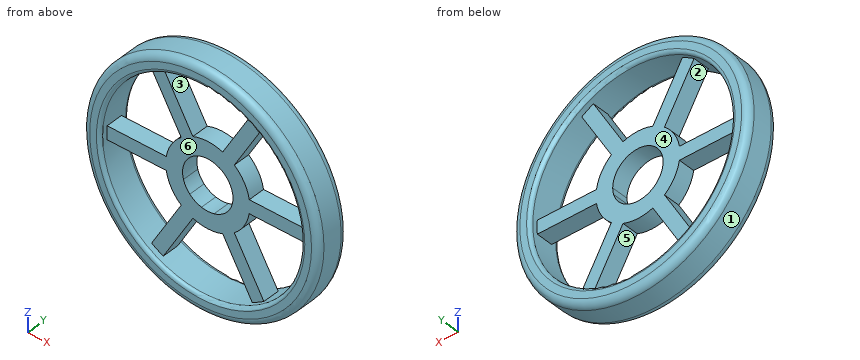
Autodesk Inventor part; units mm, degrees
ref_plane "YZ Plane" through (0, 0, 0) normal (1, 0, 0) x (0, 1, 0)
ref_plane "XZ Plane" through (0, 0, 0) normal (0, 1, 0) x (-1, 0, 0)
ref_plane "XY Plane" through (0, 0, 0) normal (0, 0, 1) x (1, 0, 0)
sketch "스케치1" plane through (0, 0, 0) normal (0, 1, 0) x (-1, 0, 0)
  circle A0 centre (0, 0) radius 37.5
  circle A1 centre (0, 0) radius 7.5
  circle A2 centre (0, 0) radius 12.5
  line L0 (2, 37.5) -> (-2, 37.5)
  line L1 (-2, 37.5) -> (-2, -37.5)
  line L2 (-2, -37.5) -> (2, -37.5)
  line L3 (2, -37.5) -> (2, 37.5)
  dimension "d0" = 75
  dimension "d1" = 15
  dimension "d2" = 25
  dimension "d3" = 2
  dimension "d4" = 2
  dimension "d5" = 75
  dimension "d6" = 37.5
extrude "돌출1" add sketch "스케치1" along normal blind 5 contours L3 A1 L1 A2 | A2 L3 A1 | A2 L1 A1 L3 | L1 A1 A2
sketch "스케치2" plane through (0, 5, 0) normal (0, 1, 0) x (1, 0, 0)
  circle A0 centre (0, 0) radius 35
  circle A1 centre (0, 0) radius 30
  dimension "d9" = 70
  dimension "d10" = 60
extrude "돌출2" add sketch "스케치2" against normal blind 7.5
sketch "스케치3" plane through (0, 5, 0) normal (0, 1, 0) x (1, 0, 0)
  circle A0 centre (0, 0) radius 30
  circle A1 centre (0, 0) radius 35
extrude "돌출3" add sketch "스케치3" along normal blind 2.5
sketch "스케치4" plane through (0, 5, 0) normal (0, 1, 0) x (1, 0, 0)
  line L0 (-34, -2) -> (34, -2)
  line L1 (34, -2) -> (34, 2)
  line L2 (34, 2) -> (-34, 2)
  line L3 (-34, 2) -> (-34, -2)
  point P0 (0, 0)
  dimension "d15" = 68
  dimension "d16" = 4
  dimension "d17" = 2
  dimension "d18" = 34
extrude "돌출4" add sketch "스케치4" against normal blind 5
pattern_circular "원형 패턴1" count 6 over 360 about axis through (0, 0, 0) along (0, 1, 0) of "돌출4"
sketch "스케치5" plane through (0, 5, 0) normal (0, 1, 0) x (1, 0, 0)
  circle A0 centre (0, 0) radius 7.5
  arc A1 (1.8822, 7.26) -> (-1.8822, 7.26) centre (0, 0) ccw
extrude "돌출5" cut sketch "스케치5" against normal blind 5
fillet "모깎기1" radius 2 2 edges at (-35, 7.5, 0) (-35, -2.5, 0)
fillet "모깎기2" radius 1 1 edges at (-30, 7.5, 0)
fillet "모깎기3" radius 1 1 edges at (-30, -2.5, 0)
properties part number "앞바퀴2"
The listing builds one solid part. Answer for the finished solid, in the listing's coordinates (mm). Face numbers are marked on the shaded views. A direction names the side the tool comes from. Round coordinates to 2 decimals unless told otherwise and drop trailing zeros. Loops run counter-clockwise (first coordinate to the right, second up) from the corner with the lowest first, then second, coordinate; pieces in that order, holes last.
Q1. Section A-A, the plane x = 0 is taken. Determine the outline of the cut face in (y, z), then the cut area to 3 significant figures.
Q2. For a pull along Z with two mould halves and no side action, classify the marked faces 1, 2 and 3 as released by +Z, released by -Z, zero draft, split by the parting line, or undercut.
Q3. Section C-C, the plane z = 14 is taken. Count the separate pieces of the cut face and the enclosed holes in it, then the cut area to 3 significant figures.
Q4. Section B-B, the plane y = 4 is taken. Determine the outline of the cut face in (x, z).
Q5. Find the intervals of material crossed by line 1 (Z direction, x = 0, y = 3.5); line 2 (X direction, y = 4.5, z = 13.5); line 3 (Z direction, x = -14.5, y = 0.75), in increasing order.
Q6. Given pin 1 Ø2 at (y, z) = (5.5, 9) entering from +X; pin 2 Ø5 at (x, y) = (-26, 1.5) entering from +Z; pin 3 Ø5 at (x, y) = (-20.5, 4) entering from +Z; pin 4 Ø8 at (x, z) = (-11.5, -26.5) entering from -Y, each flat-ended and moving along its own axis, determine where each tip first touches the part or whether it passes through.
Q7. Which of the six approach directions +Z, -Z, +X, -X, +Y, -Y give full straight-line access (tool end or side, diameter ignored) to the marked faces 4, 5 and 6?
Completed:
1. outline: (-2.5, -33) arc R2 ccw to (-0.5, -35) - (5.5, -35) arc R2 ccw to (7.5, -33) - (7.5, -31) arc R1 ccw to (6.5, -30) - (-1.5, -30) arc R1 ccw to (-2.5, -31) - close; (-2.5, 31) arc R1 ccw to (-1.5, 30) - (6.5, 30) arc R1 ccw to (7.5, 31) - (7.5, 33) arc R2 ccw to (5.5, 35) - (-0.5, 35) arc R2 ccw to (-2.5, 33) - close; (0, -12.5) - (5, -12.5) - (5, -7.5) - (0, -7.5) - close; (0, 7.5) - (5, 7.5) - (5, 12.5) - (0, 12.5) - close
1. area: 146 mm2
2. face 1: split by the parting line
2. face 2: undercut
2. face 3: undercut
3. separate pieces: 4
3. enclosed holes: 0
3. area: 152 mm2
4. outline: circle Ø70 at (0, 0); hole (-29.93, -2) arc R30 ccw to (-16.7, -24.92) - (-7.9, -9.69) arc R12.5 cw to (-12.34, -2) - close; hole (-29.93, 2) - (-12.34, 2) arc R12.5 cw to (-7.9, 9.69) - (-16.7, 24.92) arc R30 ccw to start; hole (-13.23, -26.92) arc R30 ccw to (13.23, -26.92) - (4.44, -11.69) arc R12.5 cw to (-4.44, -11.69) - close; hole (-13.23, 26.92) - (-4.44, 11.69) arc R12.5 cw to (4.44, 11.69) - (13.23, 26.92) arc R30 ccw to start; hole circle Ø15 at (0, 0); hole (7.9, -9.69) - (16.7, -24.92) arc R30 ccw to (29.93, -2) - (12.34, -2) arc R12.5 cw to start; hole (7.9, 9.69) arc R12.5 cw to (12.34, 2) - (29.93, 2) arc R30 ccw to (16.7, 24.92) - close
5. line 1: z = -35 to -30, -12.5 to -7.5, 7.5 to 12.5, 30 to 35
5. line 2: x = -32.29 to -26.79, -10.1 to -5.48, 5.48 to 10.1, 26.79 to 32.29
5. line 3: z = -31.86 to -21.11, -2 to 2, 21.11 to 31.86
6. pin 1: stops at x = 34.07
6. pin 2: stops at z = 25.94
6. pin 3: stops at z = 30.02
6. pin 4: stops at y = -2.5
7. face 4: +Y
7. face 5: +Y, -Y
7. face 6: -Y
